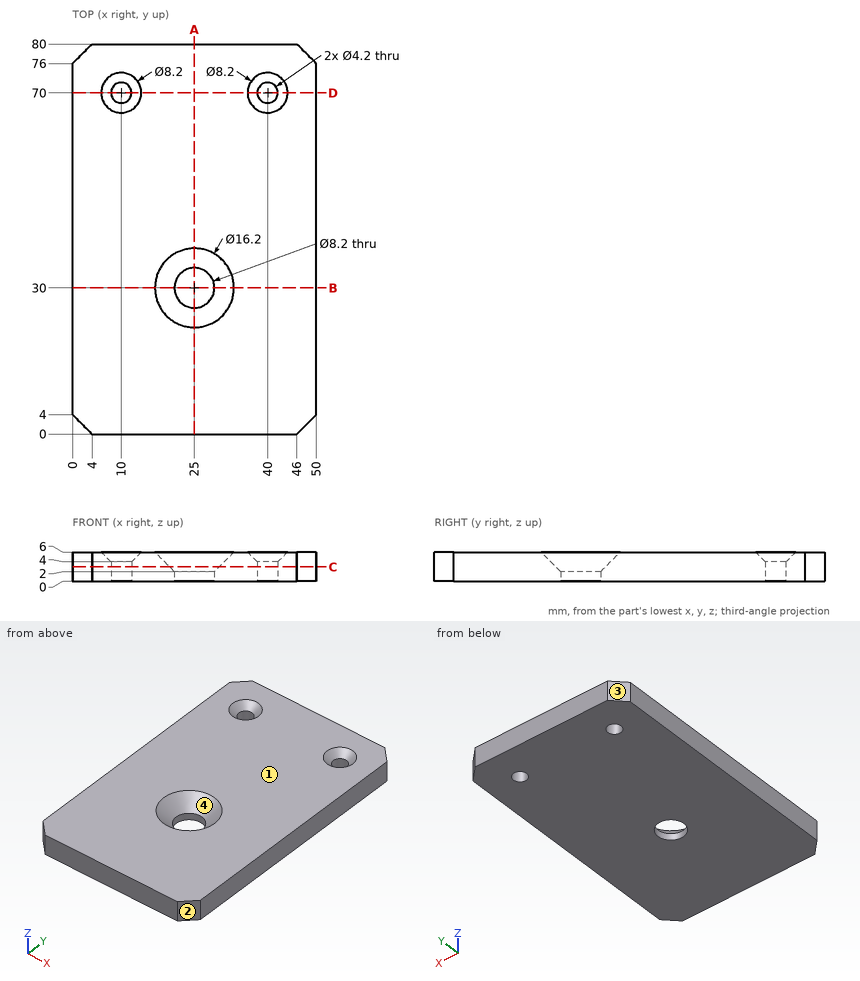
Answer from the drawing. Dimensions are ordinates in mm from the lowest x, y and z of the part. Give positions to 0.01 mm unless a question says otherwise; leave off trailing zeros. Order: outer loops, then holes, each group sorted by start corner. A loop starts at its lowest first (then second) coordinate and runs counter-clockwise, first axis right, second up. Notation, with made-up numbers: (32, -28.75) -> (69, -28.75) arc R30 ccw to (69, -4.75) -> close; hole circle Ø2 at (70.5, 1.25). An arc over 180 degrees is marked (long way). Answer as a JSON object with one key per item and string values. Group by question number.
1. The mould has two halves that part along X. Classify the marked faces 1, 2, 3 and 4: released by +X, released by -X, zero draft, split by the parting line, or undercut.
2. Section B-B on y = 30 is taken. Determine the outline of the cut face in (x, z), plus the area to 3 significant figures.
3. Section A-A on x = 25 is taken. Determine the outline of the cut face in (y, z).
4. Section C-C on z = 3 is taken. Determine the outline of the cut face in (x, y).
5. Consider line 1 along X through (y, z) = (70, 1.05); line 2 along Y through (x, z) = (40, 1.7); line 3 along X through (y, z) = (29, 3.75). Determine where each line is inside the solid, lowest interval first. Write a range as [from, to].
6. Section D-D on y = 70 is taken. Determine the outline of the cut face in (x, z), plus the area to 3 significant figures.
7. Flat-ended cylindrical pins translate along their axes: pin 1 Ø2 at (x, z) = (41.5, 3.5) entering from -Y; pin 2 Ø10.5 at (x, y) = (25, 30) entering from +Z. Find the tip coordinate at first contact, or state that the pin passes through.
Result sheet:
{
 "1": {"face 1": "zero draft", "face 2": "released by +X", "face 3": "released by -X", "face 4": "undercut"},
 "2": {"outline": "(0, 0) -> (20.9, 0) -> (20.9, 2) -> (16.9, 6) -> (0, 6) -> close; (29.1, 0) -> (50, 0) -> (50, 6) -> (33.1, 6) -> (29.1, 2) -> close", "area": "235 mm^2"},
 "3": {"outline": "(0, 0) -> (25.9, 0) -> (25.9, 2) -> (21.9, 6) -> (0, 6) -> close; (34.1, 0) -> (80, 0) -> (80, 6) -> (38.1, 6) -> (34.1, 2) -> close"},
 "4": {"outline": "(0, 4) -> (4, 0) -> (46, 0) -> (50, 4) -> (50, 76) -> (46, 80) -> (4, 80) -> (0, 76) -> close; hole circle Ø4.2 at (10, 70); hole circle Ø10.2 at (25, 30); hole circle Ø4.2 at (40, 70)"},
 "5": {"line 1": "x = [0, 7.9], [12.1, 37.9], [42.1, 50]", "line 2": "y = [0, 67.9], [72.1, 80]", "line 3": "x = [0, 19.24], [30.76, 50]"},
 "6": {"outline": "(0, 0) -> (7.9, 0) -> (7.9, 4) -> (5.9, 6) -> (0, 6) -> close; (12.1, 0) -> (37.9, 0) -> (37.9, 4) -> (35.9, 6) -> (14.1, 6) -> (12.1, 4) -> close; (42.1, 0) -> (50, 0) -> (50, 6) -> (44.1, 6) -> (42.1, 4) -> close", "area": "242 mm^2"},
 "7": {"pin 1": "stops at y = 0", "pin 2": "stops at z = 3.15"}
}
